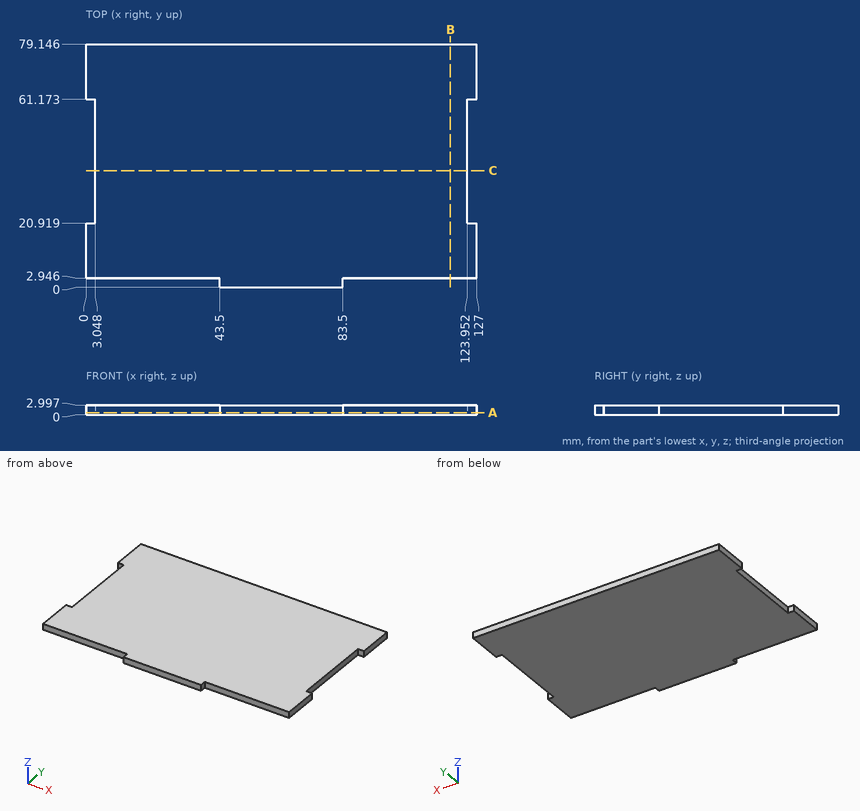
Part print with two shaded views. Sizes in mm from the minimum x, y, z corner. Round coordinates to 2 decimals unless told otherwise and drop trailing zeros. Order: outer loops, then holes, each group sorted by start corner. A loop starts at its lowest first (then second) coordinate and runs counter-clockwise, first axis right, second up. Notation, with made-up numbers: (69.5, 30.5) -> (112.5, 30.5) arc R26 cw to (112.5, 64.5) -> close; hole circle Ø1 at (11.5, 87). An arc over 180 degrees is marked (long way). Use one line per item in the form item = value.
Item 1: Drill centre lines: line 1 (X direction, y = 30, z = 1.6); line 2 (Y direction, x = 23.5, z = 1.85). Where is each one in solid material? Low to high.
Returned:
line_1 = 3.05 to 123.95
line_2 = 2.95 to 79.15
Item 2: Flat gauge pins, fed straight in: pin 1 Ø0.9 at (y, z) = (1.5, 1.5) entering from +X; pin 2 Ø1.5 at (x, z) = (2, 1.5) entering from -Y; pin 3 Ø0.9 at (y, z) = (37, 2) entering from +X. Where does each tip first touch, or does it go through?
Returned:
pin_1 = 83.5
pin_2 = 2.95
pin_3 = 123.95
Item 3: Cut at C-C, the plane y = 38. Write the cut outline in (x, z).
Returned:
outline = (3.05, 0) -> (123.95, 0) -> (123.95, 3) -> (3.05, 3) -> close
Item 4: Cut at B-B, the plane x = 118.5. Write the cut outline in (y, z).
Returned:
outline = (2.95, 0) -> (79.15, 0) -> (79.15, 3) -> (2.95, 3) -> close
Item 5: Cut at A-A, the plane z = 0.65. Write the cut outline in (x, y), and give its area (3 significant figures).
Returned:
outline = (0, 2.95) -> (43.5, 2.95) -> (43.5, 0) -> (83.5, 0) -> (83.5, 2.95) -> (127, 2.95) -> (127, 20.92) -> (123.95, 20.92) -> (123.95, 61.17) -> (127, 61.17) -> (127, 79.15) -> (0, 79.15) -> (0, 61.17) -> (3.05, 61.17) -> (3.05, 20.92) -> (0, 20.92) -> close
area = 9,550 mm^2
